Autodesk Inventor part; units mm, degrees
ref_plane "YZ Plane" through (0, 0, 0) normal (1, 0, 0) x (0, 1, 0)
ref_plane "XZ Plane" through (0, 0, 0) normal (0, 1, 0) x (-1, 0, 0)
ref_plane "XY Plane" through (0, 0, 0) normal (0, 0, 1) x (1, 0, 0)
sketch "Sketch1" plane through (0, 0, 0) normal (0, 1, 0) x (-1, 0, 0)
  line L0 (142.5, 197.5) -> (-142.5, 197.5) construction
  line L1 (-142.5, 197.5) -> (-142.5, -197.5) construction
  line L2 (-142.5, -197.5) -> (142.5, -197.5) construction
  line L3 (142.5, -197.5) -> (142.5, 197.5) construction
  line L4 (142.5, 197.5) -> (-142.5, -197.5) construction
  line L5 (-142.5, 197.5) -> (142.5, -197.5) construction
  line L6 (275, -235) -> (-275, -235) construction
  line L7 (-275, -235) -> (-275, 235) construction
  line L8 (-275, 235) -> (275, 235) construction
  line L9 (275, 235) -> (275, -235) construction
  line L10 (275, -235) -> (-275, 235) construction
  line L11 (-275, -235) -> (275, 235) construction
  line L12 (274.0052, -241.4689) -> (274.0052, -478.1407) construction
  line L13 (274.0052, -478.1407) -> (222.5538, -478.1407) construction
  line L14 (222.5538, -478.1407) -> (222.5538, -241.4689) construction
  line L15 (222.5538, -241.4689) -> (274.0052, -241.4689) construction
  line L16 (200, 212.5) -> (-200, 212.5)
  line L17 (-200, 212.5) -> (-200, 182.5)
  line L18 (-200, 182.5) -> (200, 182.5)
  line L19 (200, 182.5) -> (200, 212.5)
  line L20 (200, 212.5) -> (-200, 182.5) construction
  line L21 (-200, 212.5) -> (200, 182.5) construction
  line L22 (200, -182.5) -> (-200, -182.5)
  line L23 (-200, -182.5) -> (-200, -212.5)
  line L24 (-200, -212.5) -> (200, -212.5)
  line L25 (200, -212.5) -> (200, -182.5)
  line L26 (200, -182.5) -> (-200, -212.5) construction
  line L27 (-200, -182.5) -> (200, -212.5) construction
  circle A0 centre (142.5, 197.5) radius 4
  circle A1 centre (142.5, -197.5) radius 4
  circle A2 centre (-142.5, 197.5) radius 4
  circle A3 centre (-142.5, -197.5) radius 4
  point P0 (0, 0)
  point P1 (0, 197.5)
  point P2 (0, -197.5)
  dimension "d0" = 285
  dimension "d1" = 395
  dimension "d2" = 550
  dimension "d3" = 470
  dimension "d10" = 400
  dimension "d11" = 30
  dimension "d12" = 400
  dimension "d13" = 30
  dimension "d14" = 8
  dimension "d15" = 8
  dimension "d16" = 8
  dimension "d17" = 8
sketch "Sketch2" plane through (0, 0, 0) normal (0, 1, 0) x (-1, 0, 0)
  line L0 (142.5, 197.5) -> (-142.5, 197.5) construction
  line L1 (142.5, -197.5) -> (142.5, 197.5) construction
  line L2 (-142.5, -197.5) -> (142.5, -197.5) construction
  line L3 (-142.5, 197.5) -> (-142.5, -197.5) construction
  line L4 (250, 217.5) -> (-250, 217.5)
  line L5 (-250, 217.5) -> (-250, 177.5)
  line L6 (-250, 177.5) -> (250, 177.5)
  line L7 (250, 177.5) -> (250, 217.5)
  line L8 (250, 217.5) -> (-250, 177.5) construction
  line L9 (-250, 217.5) -> (250, 177.5) construction
  line L10 (250, -177.5) -> (-250, -177.5)
  line L11 (-250, -177.5) -> (-250, -217.5)
  line L12 (-250, -217.5) -> (250, -217.5)
  line L13 (250, -217.5) -> (250, -177.5)
  line L14 (250, -177.5) -> (-250, -217.5) construction
  line L15 (-250, -177.5) -> (250, -217.5) construction
  line L16 (250, 217.5) -> (210, 217.5)
  line L17 (210, 217.5) -> (210, -217.5)
  line L18 (210, -217.5) -> (250, -217.5)
  line L19 (250, -217.5) -> (250, 217.5)
  line L20 (-250, 217.5) -> (-210, 217.5)
  line L21 (-210, 217.5) -> (-210, -217.5)
  line L22 (-210, -217.5) -> (-250, -217.5)
  line L23 (-250, -217.5) -> (-250, 217.5)
  point P0 (0, 0)
  point P1 (0, 197.5)
  point P2 (0, -197.5)
  point P3 (210, -177.5)
  point P4 (-210, -177.5)
  point P5 (-210, 177.5)
  point P6 (210, 177.5)
  dimension "d4" = 500
  dimension "d5" = 40
  dimension "d6" = 500
  dimension "d7" = 40
  dimension "d8" = 40
  dimension "d9" = 40
extrude "Extrusion1" add sketch "Sketch2" against normal blind 40 contours L7 L6 L17 L4 | L17 L6 L21 L4 | L19 L10 L17 L6 | L21 L6 L5 L4 | L13 L12 L17 L10 | L21 L10 L23 L6 | L17 L12 L21 L10 | L21 L12 L11 L10
extrude "Extrusion2" add sketch "Sketch1" along normal blind 10
sketch "Sketch3" plane through (0, -40, 0) normal (0, -1, 0) x (1, 0, 0)
  line L0 (250, -217.5) -> (250, 217.5) construction
  line L1 (250, 217.5) -> (-250, 217.5) construction
  line L2 (-250, -217.5) -> (250, -217.5) construction
  line L3 (-250, 217.5) -> (-250, -217.5) construction
  line L4 (250, 217.5) -> (250, -217.5)
  line L5 (210, 177.5) -> (210, -177.5)
  line L6 (250, 217.5) -> (210, 217.5)
  line L7 (210, 217.5) -> (210, 177.5)
  line L8 (210, 177.5) -> (250, 177.5)
  line L9 (250, 177.5) -> (250, 217.5)
  line L10 (250, -217.5) -> (-250, -217.5)
  line L11 (210, -177.5) -> (250, -177.5)
  line L12 (250, -177.5) -> (250, -217.5)
  line L13 (250, -217.5) -> (210, -217.5)
  line L14 (210, -217.5) -> (210, -177.5)
  line L15 (-250, -217.5) -> (-210.2265, -217.5)
  line L16 (-210.2265, -217.5) -> (-210.2265, -177.5)
  line L17 (-210.2265, -177.5) -> (-250, -177.5)
  line L18 (-250, -177.5) -> (-250, -217.5)
  line L19 (-210, 177.5) -> (-210, -177.5)
  line L20 (-250, -217.5) -> (-250, 217.5)
  line L21 (-210, 177.5) -> (-250, 177.5)
  line L22 (-250, 177.5) -> (-250, 217.5)
  line L23 (-250, 217.5) -> (-210, 217.5)
  line L24 (-210, 217.5) -> (-210, 177.5)
  point P0 (0, 0)
extrude "Extrusion3" add sketch "Sketch3" along normal blind 150 contours L20 L23 L24 L21 | L10 L18 L17 L16 | L4 L8 L7 L6 | L4 L10 L14 L11
sketch "Sketch4" plane through (-250, 0, -217.5) normal (-1, 0, 0) x (0, 0, 1)
  line L0 (0, 0) -> (435, 0) construction
  line L1 (0, 0) -> (0, -190) construction
  line L2 (40, -190) -> (0, -190) construction
  line L3 (40, -40) -> (40, -190) construction
  line L4 (395, -40) -> (40, -40) construction
  line L5 (395, -40) -> (395, -190) construction
  line L6 (435, -190) -> (395, -190) construction
  line L7 (435, 0) -> (435, -190) construction
  line L8 (0, -40) -> (0, -190)
  line L9 (40, -40) -> (40, -190)
  line L10 (0, -190) -> (40, -190)
  line L11 (40, -190) -> (40, -150)
  line L12 (40, -150) -> (0, -150)
  line L13 (0, -150) -> (0, -190)
  line L14 (395, -40) -> (395, -190)
  line L15 (435, 0) -> (435, -190)
  line L16 (395, -190) -> (435, -190)
  line L17 (435, -190) -> (435, -150)
  line L18 (435, -150) -> (395, -150)
  line L19 (395, -150) -> (395, -190)
  point P0 (217.5, 0)
  dimension "d24" = 40
  dimension "d25" = 40
extrude "Extrusion4" add sketch "Sketch4" along normal blind 500
sketch "Sketch5" plane through (-250, -40, -177.5) normal (0, 0, 1) x (1, 0, 0)
  line L0 (0, 0) -> (39.7735, 0) construction
  line L1 (0, 0) -> (0, -110) construction
  line L2 (0, -110) -> (-500, -110) construction
  line L3 (-500, -150) -> (-500, -110) construction
  line L4 (39.7735, -150) -> (-500, -150) construction
  line L5 (39.7735, 0) -> (39.7735, -150) construction
  line L6 (0, -110) -> (-500, -110)
  line L7 (-500, -110) -> (-460, -110)
  line L8 (-460, -110) -> (-460, -150)
  line L9 (-460, -150) -> (-500, -150)
  line L10 (-500, -150) -> (-500, -110)
  point P0 (250, 40)
  dimension "d28" = 40
  dimension "d29" = 40
extrude "Extrusion5" add sketch "Sketch5" along normal up to surface (355 mm away)
sketch "Sketch6" plane through (-250, -150, 217.5) normal (0, 1, 0) x (1, 0, 0)
  line L0 (0, 40) -> (0, 0) construction
  line L1 (0, 40) -> (-460, 40) construction
  line L2 (-460, 395) -> (-460, 40) construction
  line L3 (0, 395) -> (-460, 395) construction
  line L4 (0, 435) -> (0, 395) construction
  line L5 (0, 435) -> (-500, 435) construction
  line L6 (-500, 0) -> (-500, 435) construction
  line L7 (0, 0) -> (-500, 0) construction
  line L8 (-460, 0) -> (-760, 0)
  line L9 (-760, 0) -> (-760, 435)
  line L10 (-760, 435) -> (-460, 435)
  line L11 (-460, 435) -> (-460, 0)
  point P0 (250, 217.5)
  dimension "d32" = 300
extrude "Extrusion6" add sketch "Sketch6" along normal blind 3
sketch "Sketch7" plane through (-710, -190, -177.5) normal (1, 0, 0) x (0, 0, -1)
  line L0 (-355, 0) -> (-355, 40) construction
  line L1 (0, 0) -> (-355, 0) construction
  line L2 (0, 40) -> (0, 0) construction
  line L3 (40, 40) -> (0, 40) construction
  line L4 (40, 40) -> (40, 43) construction
  line L5 (-395, 43) -> (40, 43) construction
  line L6 (-395, 40) -> (-395, 43) construction
  line L7 (-355, 40) -> (-395, 40) construction
  line L8 (-197.5, 40) -> (-157.5, 40)
  line L9 (-157.5, 40) -> (-157.5, 0)
  line L10 (-157.5, 0) -> (-197.5, 0)
  line L11 (-197.5, 0) -> (-197.5, 40)
  line L12 (-197.5, 40) -> (-157.5, 0) construction
  line L13 (-157.5, 40) -> (-197.5, 0) construction
  point P0 (-177.5, 190)
  point P1 (-177.5, 20)
  dimension "d35" = 40
  dimension "d36" = 40
extrude "Extrusion7" add sketch "Sketch7" along normal blind 200
properties part number "test1"
CAD build for the part. Positions are in the model's coordinates, mm. A direction names the side the tool comes from. Round coordinates to 2 decimals unless told otherwise and drop trailing zeros. Loops run counter-clockwise (first coordinate to the right, second up) from the corner with the lowest first, then second, coordinate; pieces in that order, holes last. Notation, with made-up numbers: M 47.5,62 L 98.5,62 A16 cw 98.5,67 Z; hole C 16,-30.5 d11. An arc over 180 degrees is marked long. Use a Markdown table: item, result. Add a question column.
(1) Cut at B-B (y = -161). Give the cut face in (x, z).
(2) Cut at D-D (y = -78.5). Give the cut face in (x, z), and give its area (3 significant figures).
(3) Cut at C-C (x = -474.5). Give the cut face in (y, z).
(4) Which spindle directions (+Z, -Z, +X, -X, +Y, -Y) get a long thin tool onto all of the face, cutting with end or side? Do faces 4 (the face through (-882, -150, -3)), 5 (the face through (-210, -114, 198)), 6 (the face through (230, -114, 177.5)), 7 (the face through (-862, -147, -3)), 8 (the face through (-210, -20, 2)). Say none if no direction does.
(5) Cut at A-A (z = 145). Give the cut face in (x, y), and give its area (3 significant figures).
(6) Flat gauge pins, fed straight in: pin 1 (11 mm diameter, centred on x = 33.5, y = 6, fed in from +Z); pin 2 (10 mm diameter, centred on y = -165, z = -43, fed in from +X); pin 3 (3 mm diameter, centred on y = 3.5, z = 191.5, fed in from -X). Where does each tip first touch, or does it go through?
(7) Drill centre lines: line 1 (X direction, y = 5, z = 197); line 2 (Z direction, x = -578, y = -160.5); line 3 (Z direction, x = 142.5, y = 6.75). Where is each one in solid material? Low to high.
(8) Pull direction Z, two halves, no side cores. Call faces 1 (the face through (-559, -190, -17)), 2 (the face through (-510, -170, 0)), 3 (the face through (-243, -95, -217.5)): +Z half, -Z half, draft (parallel to the pull), parting line (faces both ways), or undercut.
Geometry says:
| question | item | result |
|---|---|---|
| 1 | outline | M -750,-217.5 L -210.23,-217.5 L -210.23,-177.5 L -710,-177.5 L -710,-20 L -510,-20 L -510,20 L -710,20 L -710,177.5 L -210,177.5 L -210,217.5 L -750,217.5 Z; M 210,-217.5 L 250,-217.5 L 250,-177.5 L 210,-177.5 Z; M 210,177.5 L 250,177.5 L 250,217.5 L 210,217.5 Z |
| 2 | outline | M -250,-217.5 L -210.23,-217.5 L -210.23,-177.5 L -250,-177.5 Z; M -250,177.5 L -210,177.5 L -210,217.5 L -250,217.5 Z; M 210,-217.5 L 250,-217.5 L 250,-177.5 L 210,-177.5 Z; M 210,177.5 L 250,177.5 L 250,217.5 L 210,217.5 Z |
| 2 | area | 6,390 mm² |
| 3 | outline | M -190,-217.5 L -150,-217.5 L -150,-177.5 L -190,-177.5 Z; M -190,177.5 L -150,177.5 L -150,217.5 L -190,217.5 Z |
| 4 | face 4 | +Z, -Z, -X, -Y |
| 4 | face 5 | +Z, -Z, -Y |
| 4 | face 6 | +X, -Y |
| 4 | face 7 | +Z, -Z, -X, +Y |
| 4 | face 8 | +Y, -Y |
| 5 | outline | M -1010,-150 L -750,-150 L -750,-190 L -710,-190 L -710,-147 L -1010,-147 Z; M -250,-40 L -210,-40 L -210,0 L -250,0 Z; M 210,-40 L 250,-40 L 250,0 L 210,0 Z |
| 5 | area | 5,700 mm² |
| 6 | pin 1 | stops at z = 212.5 |
| 6 | pin 2 | stops at x = -710 |
| 6 | pin 3 | stops at x = -200 |
| 7 | line 1 | x = -200 to -146.47, -138.53 to 138.53, 146.47 to 200 |
| 7 | line 2 | z = -217.5 to -177.5, -20 to 20, 177.5 to 217.5 |
| 7 | line 3 | z = -212.5 to -201.5, -193.5 to -182.5, 182.5 to 193.5, 201.5 to 212.5 |
| 8 | face 1 | draft |
| 8 | face 2 | undercut |
| 8 | face 3 | -Z half |
